Input: part model. Units: mm. Frame: model coordinates. A direction names the side the tool comes from. Give positions to 0.01 mm unless a question says otherwise; leave off trailing zeros. Write each loop counter-clockwise with the first axis right and the second up, starting at its lowest first coordinate (ties: lowest second). Pieces come first, ordered by that corner, then holes.
```python
from build123d import *

# Parameters (mm, degrees)
BOSS_EXTRUDE1_DEPTH      = 5
BOSS_EXTRUDE1_DEPTH_BACK = 9
SKETCH1_W                = 53
SKETCH1_H                = 88
BOSS_EXTRUDE3_DEPTH      = 2
SKETCH7_W                = 49
SKETCH7_H                = 3
CUT_EXTRUDE3_DEPTH       = 75.934971809
LPATTERN1_COUNT          = 11
LPATTERN1_PITCH          = 8


with BuildPart() as part:
    # Sketch1 → Boss-Extrude1 (new, two sides: drawn at the far end of the back side and taken through both)
    with BuildSketch(Plane(origin=(0, 15, 0), x_dir=(1, 0, 0), z_dir=(0, 1, 0)).offset(-BOSS_EXTRUDE1_DEPTH_BACK)):
        with BuildLine():
            Line((29.5, -65), (29.5, 25))
            ThreePointArc((29.5, 25), (28.914213562, 26.414213562), (27.5, 27))
            Line((27.5, 27), (-27.5, 27))
            ThreePointArc((-27.5, 27), (-28.914213562, 26.414213562), (-29.5, 25))
            Line((-29.5, 25), (-29.5, -65))
            ThreePointArc((-29.5, -65), (-28.914213562, -66.414213562), (-27.5, -67))
            Line((-27.5, -67), (27.5, -67))
            ThreePointArc((27.5, -67), (28.914213562, -66.414213562), (29.5, -65))
        make_face()
        with Locations((0, -20)):
            Rectangle(SKETCH1_W, SKETCH1_H, mode=Mode.SUBTRACT)
    extrude(amount=BOSS_EXTRUDE1_DEPTH + BOSS_EXTRUDE1_DEPTH_BACK)

    # Sketch2 → Boss-Extrude3 (add)
    with BuildSketch(Plane(origin=(0, 20, 0), x_dir=(1, 0, 0), z_dir=(0, 1, 0))):
        with BuildLine():
            Line((29.5, -65), (29.5, 25))
            ThreePointArc((29.5, 25), (28.914213562, 26.414213562), (27.5, 27))
            Line((27.5, 27), (-27.5, 27))
            ThreePointArc((-27.5, 27), (-28.914213562, 26.414213562), (-29.5, 25))
            Line((-29.5, 25), (-29.5, -65))
            ThreePointArc((-29.5, -65), (-28.914213562, -66.414213562), (-27.5, -67))
            Line((-27.5, -67), (27.5, -67))
            ThreePointArc((27.5, -67), (28.914213562, -66.414213562), (29.5, -65))
        make_face()
    extrude(amount=BOSS_EXTRUDE3_DEPTH)

    # Sketch7 → Cut-Extrude3 (cut, through all)
    with BuildSketch(Plane(origin=(0, 22, 0), x_dir=(1, 0, 0), z_dir=(0, 1, 0))):
        with Locations((0, 20.5)):
            Rectangle(SKETCH7_W, SKETCH7_H)
    cut_extrude3 = extrude(amount=-CUT_EXTRUDE3_DEPTH, mode=Mode.SUBTRACT)

    # LPattern1: Cut-Extrude3 ×11
    with Locations(*[(0, 0, i * LPATTERN1_PITCH) for i in range(1, LPATTERN1_COUNT)]):
        add(cut_extrude3, mode=Mode.SUBTRACT)


solid = part.part
```
Q1. Section D-D, the plane x = -4.5. Give the number of separate pieces and of enclosed holes in the cut face, then the cut area to 3 significant figures.
Q2. Section C-C, the plane z = -7. Return the cut outline in (x, y).
Q3. Section B-B, the plane y = 15.75. Return the cut outline in (x, z).
Q4. Access query for faces 1 (the flat face through (-0.4, 20, 9.6)), 2 (the flat face through (0, 21, 50)). Directions: +Z, -Z, +X, -X, +Y, -Y. A direction counts if a zero-diameter tool reaches every point of the face in a straight line with its end or side. Return the directions, or none.
Q5. Mould query, pull axis Z, two halves, no side actions, for faces 3 (the cylindrical face through (28.9, 13.89, 66.43)), 4 (the flat face through (0, 21, 58)). Classes: +Z half, -Z half, draft (parallel to the pull), parting line (faces both ways), or undercut.
Q6. Material intervals for line 1 along Z through (x, y) = (8, 11); line 2 along X through (y, z) = (16, 25); line 3 along Y through (x, z) = (-8, 41.5), sorted ascending.
Q7. Section A-A, the plane z = 19.5. Return the cut outline in (x, y), then the cut area to 3 significant figures.
Solutions:
1. separate pieces: 12
1. enclosed holes: 0
1. area: 206 mm2
2. outline: (-29.5, 6) - (-26.5, 6) - (-26.5, 20) - (26.5, 20) - (26.5, 6) - (29.5, 6) - (29.5, 22) - (-29.5, 22) - close
3. outline: (-29.5, -25) arc R2 ccw to (-27.5, -27) - (27.5, -27) arc R2 ccw to (29.5, -25) - (29.5, 65) arc R2 ccw to (27.5, 67) - (-27.5, 67) arc R2 ccw to (-29.5, 65) - close; hole (-26.5, -24) - (26.5, -24) - (26.5, 64) - (-26.5, 64) - close
4. face 1: -Y
4. face 2: +Y, -Y
5. face 3: +Z half
5. face 4: undercut
6. line 1: z = -27 to -24, 64 to 67
6. line 2: x = -29.5 to -26.5, 26.5 to 29.5
6. line 3: y = 20 to 22
7. outline: (-29.5, 6) - (-26.5, 6) - (-26.5, 20) - (-24.5, 20) - (-24.5, 22) - (-29.5, 22) - close; (24.5, 20) - (26.5, 20) - (26.5, 6) - (29.5, 6) - (29.5, 22) - (24.5, 22) - close
7. area: 104 mm2
